Autodesk Inventor part; units mm, degrees
ref_plane "YZ Plane" through (0, 0, 0) normal (1, 0, 0) x (0, 1, 0)
ref_plane "XZ Plane" through (0, 0, 0) normal (0, 1, 0) x (-1, 0, 0)
ref_plane "XY Plane" through (0, 0, 0) normal (0, 0, 1) x (1, 0, 0)
sketch "Sketch2" plane through (0, 0, 0) normal (0, 0, 1) x (1, 0, 0)
  line L0 (18.75, -31.25) -> (18.75, 31.25)
  line L1 (18.75, 31.25) -> (-18.75, 31.25)
  line L2 (-18.75, 31.25) -> (-18.75, -31.25)
  line L3 (-18.75, -31.25) -> (18.75, -31.25)
  circle A0 centre (-0.1179, 25) radius 3.25
  circle A1 centre (-0.1179, -25) radius 3.25
  point P0 (0, 0)
extrude "Extrusion1" add sketch "Sketch2" along normal blind 10
sketch "Sketch4" plane through (0, 0, 10) normal (0, 0, 1) x (1, 0, 0)
  circle A0 centre (11.5, 16) radius 2.25
  circle A1 centre (-12.5, 9) radius 2.75
  circle A2 centre (-12.5, -5) radius 2.75
  circle A3 centre (11.5, -16) radius 2.25
  circle A4 centre (11.5, 16) radius 1.75
  circle A5 centre (11.5, -16) radius 1.75
  circle A6 centre (-12.5, -5) radius 1.75
  circle A7 centre (-12.5, 9) radius 1.75
  point P0 (0, 0)
  dimension "d6" = 3.5
  dimension "d7" = 3.5
  dimension "d8" = 3.5
  dimension "d9" = 3.5
  dimension "d10" = 4.5
  dimension "d11" = 4.5
  dimension "d12" = 5.5
  dimension "d13" = 5.5
extrude "Extrusion2" add sketch "Sketch4" along normal blind 1 contours A0 | A3
extrude "Extrusion3" add sketch "Sketch4" along normal blind 9 contours A1 | A2
thread "Thread1"
thread "Thread2"
thread "Thread3"
thread "Thread4"
properties part number "phm_top"
Can you work these out from the model? Positions are in its coordinate system, mm. A direction names the side the tool comes from. Coordinates: 2 decimals unless noted, no trailing zeros. Order: outer loops, then holes, each group sorted by start corner. A loop starts at its lowest first (then second) coordinate and runs counter-clockwise, first axis right, second up. Notation, with made-up numbers: M -13,12 L 40,12 A28 ccw 40,44 Z; hole C 85,51 d6. An arc over 180 degrees is marked long. Answer as CSV lines item,"result".
(1) I'm going to push flat-ended pins straight in: pin 1 (4 mm diameter, centred on x = -12.5, y = 9, fed in from +Z); pin 2 (1 mm diameter, centred on x = -13, y = -4, fed in from +Z); pin 3 (3.5 mm diameter, centred on x = 12, y = 17, fed in from +Z); pin 4 (4 mm diameter, centred on y = 6, z = 15, fed in from +X). Where does each tip first touch, or does it pass through?
Geometry check:
pin 1,"z = 19"
pin 2,"z = 10"
pin 3,"z = 11"
pin 4,"x = -9.94"
(2) Suppose I cut it at A-A on y = -25. Please give me the cut outline in (x, z).
Geometry check:
outline,"M -18.75,0 L -3.37,0 L -3.37,10 L -18.75,10 Z; M 3.13,0 L 18.75,0 L 18.75,10 L 3.13,10 Z"
(3) Please list where these lines run through material, in increasing order: L1, parallel to Y at x = -12.5, z = 12; L2, parallel to Y at x = 11.5, z = 10.6; L3, parallel to Z at x = -16.5, y = 11.
Geometry check:
L1,"-7.75 to -6.75, -3.25 to -2.25, 6.25 to 7.25, 10.75 to 11.75"
L2,"-18.25 to -17.75, -14.25 to -13.75, 13.75 to 14.25, 17.75 to 18.25"
L3,"0 to 10"
(4) If we mould it in two halves opening along X, with no side actions, what happens to faces 1 (the cylindrical face through (-9.96, 10.05, 14.44)), 2 (the flat face through (18.75, 0, 5)), 3 (the cylindrical face through (11.272, 14.265, 10.493))? For each: released by +X, released by -X, zero draft, split by the parting line, or undercut.
Geometry check:
face 1,"split by the parting line"
face 2,"released by +X"
face 3,"undercut"
(5) On a 3-axis mill with a long thin cutter (end or side, diameter ignored), from which of +Z, -Z, +X, -X, +Y, -Y can I reach the whole of each face in a straight line? I mean faces 4 (the flat face through (11, -18, 11)), 5 (the cylindrical face through (11.272, -17.735, 10.493)). Say none if no direction works.
Geometry check:
face 4,"+Z, +X, -X, +Y, -Y"
face 5,"+Z"
(6) Suppose I cut it at D-D on y = 16. Please give me the cut outline in (x, z), plus the area to 3 significant figures.
Geometry check:
outline,"M -18.75,0 L 18.75,0 L 18.75,10 L 13.75,10 L 13.75,11 L 13.25,11 L 13.25,10 L 9.75,10 L 9.75,11 L 9.25,11 L 9.25,10 L -18.75,10 Z"
area,"376 mm^2"
(7) Suppose I cut it at C-C on x = -1. Please give me the cut outline in (y, z), plus the area to 3 significant figures.
Geometry check:
outline,"M -31.25,0 L -28.13,0 L -28.13,10 L -31.25,10 Z; M -21.87,0 L 21.87,0 L 21.87,10 L -21.87,10 Z; M 28.13,0 L 31.25,0 L 31.25,10 L 28.13,10 Z"
area,"500 mm^2"
(8) Suppose I cut it at B-B on z = 14.25. Please give me the cut outline in (x, y), plus the area to 3 significant figures.
Geometry check:
outline,"C -12.5,-5 d5.5; C -12.5,9 d5.5; hole C -12.5,-5 d3.5; hole C -12.5,9 d3.5"
area,"28.3 mm^2"
